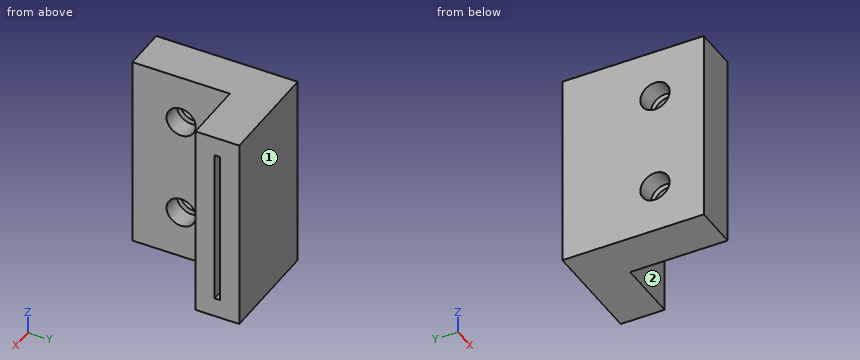
from build123d import *

# Parameters (mm, degrees)
F1_DEPTH = 40
F3_T     = -3.95
F4_D     = 6


with BuildPart() as f1:
    # F0 (on Top) → F1 (new body)
    with BuildSketch(Plane.XY):
        Polygon((-9, 0), (0, 0), (0, 20), (13, 20), (13, 29), (-9, 29), (-9, 20), align=None)
    extrude(amount=F1_DEPTH)

    # F3
    f3_openings = [f1.faces().sort_by_distance(p)[0] for p in [
        (13, 24.5, 20),
    ]]
    offset(amount=F3_T, openings=f3_openings, kind=Kind.INTERSECTION)

    # F4 (through all)
    with Locations(Plane.YZ):
        with Locations((10, 30.0820767879), (10, 9.8383650184)):
            Hole(F4_D / 2)


solid = f1.part
Here's how the part is built. I have some questions about the finished solid (model axes, mm). Face numbers are marked on the shaded views. A direction names the side the tool comes from. Coordinates: 2 decimals unless noted, no trailing zeros. Order: outer loops, then holes, each group sorted by start corner. A loop starts at its lowest first (then second) coordinate and runs counter-clockwise, first axis right, second up. Notation, with made-up numbers: (49, 28) -> (66, 28) arc R23 cw to (66, 36) -> close; hole circle Ø8 at (-13, -28.75). An arc over 180 degrees is marked (long way). Answer in a Markdown table with one row per item.
(1) On a 3-axis mill with a long thin cutter (end or side, diameter ignored), from which of +Z, -Z, +X, -X, +Y, -Y can I reach the whole of each face in a straight line? I mean the marked faces 1 and 2. Say none if no direction works.
Answer key:
| item | result |
|---|---|
| face 1 | +Z, -Z, +X, -X, +Y |
| face 2 | +Z, -Z, +X, -Y |
(2) I want a section at C-C on x = 6. List the corners of the cut face in (y, z) for me.
Answer key:
| item | result |
|---|---|
| outline | (20, 0) -> (29, 0) -> (29, 40) -> (20, 40) -> close; hole (23.95, 3.95) -> (25.05, 3.95) -> (25.05, 36.05) -> (23.95, 36.05) -> close |
(3) I want a section at D-D on y = 10. List the corners of the cut face in (x, z) for me.
Answer key:
| item | result |
|---|---|
| outline | (-9, 0) -> (0, 0) -> (0, 6.84) -> (-3.95, 6.84) -> (-3.95, 3.95) -> (-5.05, 3.95) -> (-5.05, 6.84) -> (-9, 6.84) -> close; (-9, 12.84) -> (-5.05, 12.84) -> (-5.05, 27.08) -> (-9, 27.08) -> close; (-9, 33.08) -> (-5.05, 33.08) -> (-5.05, 36.05) -> (-3.95, 36.05) -> (-3.95, 33.08) -> (0, 33.08) -> (0, 40) -> (-9, 40) -> close; (-3.95, 12.84) -> (0, 12.84) -> (0, 27.08) -> (-3.95, 27.08) -> close |
(4) Will these pins go through, and if not, where does the flat tip stop? pin 1 Ø7 at (y, z) = (10, 9.84) entering from +X; pin 2 Ø10.5 at (x, z) = (6, 21) entering from -Y; pin 3 Ø3.5 at (y, z) = (10, 9.84) entering from -X.
Answer key:
| item | result |
|---|---|
| pin 1 | x = 0 |
| pin 2 | y = 20 |
| pin 3 | through |
(5) I want a section at B-B on z = 26. List the corners of the cut face in (x, y) for me, then the cut area to 3 significant figures.
Answer key:
| item | result |
|---|---|
| outline | (-9, 0) -> (0, 0) -> (0, 20) -> (13, 20) -> (13, 23.95) -> (-3.95, 23.95) -> (-3.95, 3.95) -> (-5.05, 3.95) -> (-5.05, 25.05) -> (13, 25.05) -> (13, 29) -> (-9, 29) -> close |
| area | 336 mm^2 |
(6) Please list where these lines run through material, in increasing order: probe 1 along Z at (x, y) = (-8.05, 10); probe 2 along Y at (x, z) = (-0.5, 10); probe 3 along X at (y, z) = (17.75, 10).
Answer key:
| item | result |
|---|---|
| probe 1 | 0 to 6.84, 12.84 to 27.08, 33.08 to 40 |
| probe 2 | 0 to 7, 13 to 23.95, 25.05 to 29 |
| probe 3 | -9 to -5.05, -3.95 to 0 |
(7) I want a section at A-A on y = 14.75. List the corners of the cut face in (x, z) for me, then the cut area to 3 significant figures.
Answer key:
| item | result |
|---|---|
| outline | (-9, 0) -> (0, 0) -> (0, 40) -> (-9, 40) -> close; hole (-5.05, 3.95) -> (-3.95, 3.95) -> (-3.95, 36.05) -> (-5.05, 36.05) -> close |
| area | 325 mm^2 |
